Can you work these out from the drawing? Everything is in mm from the part's minimum corner. A direction names the side the tool comes from. Round coordinates to 2 decimals unless told otherwise and drop trailing zeros. Write each loop counter-clockwise with the first axis right and the second up, starting at its lowest first coordinate (ties: lowest second). Pieces come first, ordered by that corner, then holes. Notation, with made-up numbers: (40, -15) - (68, -15) arc R27 ccw to (68, 14) - close; hole circle Ø1 at (54, 25). An arc over 180 degrees is marked (long way). One line per item, written item: value. Start each with the question number.
Item 1: If I drill on line 1 (Z direction, x = 28, y = 2.25); line 2 (Y direction, x = 3, z = 8); line 3 (Z direction, x = 5, y = 0.6), over which ranges is the centre line in solid material (lowest first)?
Item 2: Thinking about a two-plate mould opening in Z: for the marked faces 1, 2 and 3, which applies, released by +Z, released by -Z, zero draft, split by the parting line, or undercut?
Item 3: Imagine slicing it at B-B, the plane y = 16. Please give me the cut outline in (x, z), then the cut area to 3 significant figures.
Item 4: For the marked faces 4 and 5, which set-ups out of +Z, -Z, +X, -X, +Y, -Y let a thin tool reach every point of the face, with its end or its side?
Item 5: Imagine slicing it at D-D, the plane y = 4. Please give me the cut outline in (x, z), then the cut area to 3 significant figures.
Item 6: Imagine slicing it at A-A, the plane x = 20. Please give me the cut outline in (y, z).
Item 7: Imagine slicing it at C-C, the plane z = 5.25. Please give me the cut outline in (x, y), then the cut area to 3 significant figures.
Item 8: For P1, Ø4, axis at y = 19, z = 6.5, coming from the +X side; P2, Ø1.1, axis at y = 5.5, z = 8.5, coming from the +X side; P3, Ø4.5, axis at x = 3, z = 5.5, coming from the +Y side, each with a flat end and sliding along its axis, tell me the tip position at first contact or that it passes through.
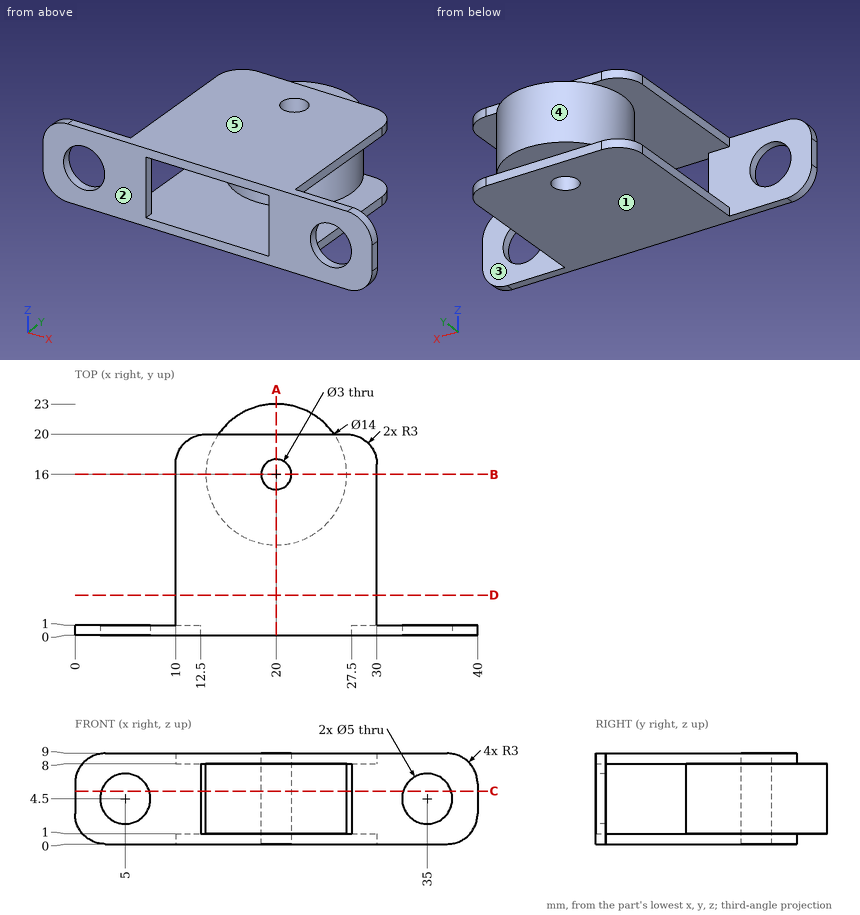
Values follow:
1. line 1: z = 0 to 1, 8 to 9
1. line 2: y = 0 to 1
1. line 3: z = 0 to 2, 7 to 9
2. face 1: released by -Z
2. face 2: zero draft
2. face 3: undercut
3. outline: (10, 0) - (18.5, 0) - (18.5, 9) - (10, 9) - (10, 8) - (13, 8) - (13, 1) - (10, 1) - close; (21.5, 0) - (30, 0) - (30, 1) - (27, 1) - (27, 8) - (30, 8) - (30, 9) - (21.5, 9) - close
3. area: 111 mm^2
4. face 4: none
4. face 5: +Z, +X, -X, +Y, -Y
5. outline: (10, 0) - (30, 0) - (30, 1) - (10, 1) - close; (10, 8) - (30, 8) - (30, 9) - (10, 9) - close
5. area: 40.0 mm^2
6. outline: (0, 0) - (14.5, 0) - (14.5, 9) - (0, 9) - (0, 8) - (9, 8) - (9, 1) - (0, 1) - close; (17.5, 0) - (20, 0) - (20, 1) - (23, 1) - (23, 8) - (20, 8) - (20, 9) - (17.5, 9) - close
7. outline: (0, 0) - (2.62, 0) - (2.62, 1) - (0, 1) - close; (7.38, 0) - (12.5, 0) - (12.5, 1) - (7.38, 1) - close; circle Ø14 at (20, 16); (27.5, 0) - (32.62, 0) - (32.62, 1) - (27.5, 1) - close; (37.38, 0) - (40, 0) - (40, 1) - (37.38, 1) - close; hole circle Ø3 at (20, 16)
7. area: 162 mm^2
8. P1: stops at x = 29.92
8. P2: stops at x = 30
8. P3: stops at y = 1
